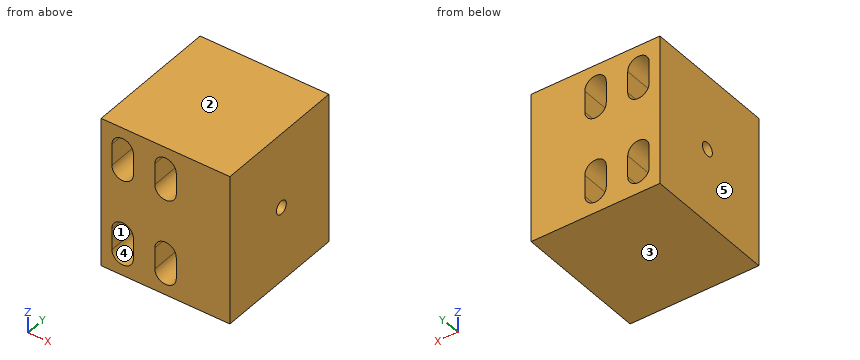
from build123d import *

# Parameters (mm, degrees)
SKETCH1_W           = 24
SKETCH1_H           = 28
BOSS_EXTRUDE1_DEPTH = 25
SKETCH2_R           = 1.25
CUT_EXTRUDE1_DEPTH  = 45.55333882


with BuildPart() as part:
    # Sketch1 → Boss-Extrude1 (new body)
    with BuildSketch(Plane(origin=(0, 0, 0), x_dir=(1, 0, 0), z_dir=(0, 1, 0))):
        with Locations((12, 14)):
            Rectangle(SKETCH1_W, SKETCH1_H)
        with BuildLine():
            Line((2, 4), (2, 8))
            ThreePointArc((2, 8), (4, 10), (6, 8))
            Line((6, 8), (6, 4))
            ThreePointArc((6, 4), (4, 2), (2, 4))
        make_face(mode=Mode.SUBTRACT)
        with BuildLine():
            Line((10, 4), (10, 8))
            ThreePointArc((10, 8), (12, 10), (14, 8))
            Line((14, 8), (14, 4))
            ThreePointArc((14, 4), (12, 2), (10, 4))
        make_face(mode=Mode.SUBTRACT)
        with BuildLine():
            Line((10, 20), (10, 24))
            ThreePointArc((10, 24), (12, 26), (14, 24))
            Line((14, 24), (14, 20))
            ThreePointArc((14, 20), (12, 18), (10, 20))
        make_face(mode=Mode.SUBTRACT)
        with BuildLine():
            Line((2, 20), (2, 24))
            ThreePointArc((2, 24), (4, 26), (6, 24))
            Line((6, 24), (6, 20))
            ThreePointArc((6, 20), (4, 18), (2, 20))
        make_face(mode=Mode.SUBTRACT)
    extrude(amount=BOSS_EXTRUDE1_DEPTH)

    # Sketch2 → Cut-Extrude1 (cut, through all)
    with BuildSketch(Plane(origin=(24, 0, 0), x_dir=(0, 0, -1), z_dir=(1, 0, 0))):
        with Locations((14, 13)):
            Circle(SKETCH2_R)
    extrude(amount=-CUT_EXTRUDE1_DEPTH, mode=Mode.SUBTRACT)


solid = part.part
For this review, take the finished solid that the model builds, in its own axes (mm). Face numbers are marked on the shaded views. A direction names the side the tool comes from. Coordinates: 2 decimals unless noted, no trailing zeros. Loops run counter-clockwise (first coordinate to the right, second up) from the corner with the lowest first, then second, coordinate; pieces in that order, holes last. Notation, with made-up numbers: (86.5, 17.5) - (92.5, 17.5) arc R14 ccw to (92.5, 37.5) - close; hole circle Ø10 at (69.25, 71). An arc over 180 degrees is marked (long way). Return JSON: item names as keys, results as strings.
Item 1: For the marked faces 1 and 2, list the 3-axis set-ups (+Z, -Z, +X, -X, +Y, -Y) from which the entire face can be reached by the end or side of a thin tool; tool diameter is ignored.
Determined:
{"face 1": "+Y, -Y", "face 2": "+Z, +X, -X, +Y, -Y"}
Item 2: Take a section at D-D (z = -19). Give the boundary of the cut face in (x, y), then the cut area to 3 significant figures.
Determined:
{"outline": "(0, 0) - (2.27, 0) - (2.27, 25) - (0, 25) - close; (5.73, 0) - (10.27, 0) - (10.27, 25) - (5.73, 25) - close; (13.73, 0) - (24, 0) - (24, 25) - (13.73, 25) - close", "area": "427 mm2"}
Item 3: Mouldability with a two-part tool opening along X and no side actions: class the marked faces 3, 4 and 5 as pulls with the +X half, pulls with the -X half, needs draft (parallel to the pull), parting line crosses it, or undercut.
Determined:
{"face 3": "needs draft", "face 4": "undercut", "face 5": "pulls with the -X half"}
Item 4: Take a section at B-B (x = 4). Give the boundary of the cut face in (y, z).
Determined:
{"outline": "(0, -28) - (25, -28) - (25, -26) - (0, -26) - close; (0, -18) - (25, -18) - (25, -10) - (0, -10) - close; (0, -2) - (25, -2) - (25, 0) - (0, 0) - close; hole circle Ø2.5 at (13, -14)"}
Item 5: Take a section at C-C (z = -14). Give the boundary of the cut face in (x, y).
Determined:
{"outline": "(0, 0) - (24, 0) - (24, 11.75) - (0, 11.75) - close; (0, 14.25) - (24, 14.25) - (24, 25) - (0, 25) - close"}
Item 6: For line 1 (X direction, y = 16.75, z = -6.5); line 2 (X direction, y = 8.5, z = -9.75); line 3 (Z direction, x = 3.5, y = 9.5), list the stretches that pass through material, from the lowest coordinate up.
Determined:
{"line 1": "x = 0 to 2, 6 to 10, 14 to 24", "line 2": "x = 0 to 3.03, 4.97 to 11.03, 12.97 to 24", "line 3": "z = -28 to -25.94, -18.06 to -9.94, -2.06 to 0"}
Item 7: Take a section at A-A (y = 13). Give the boundary of the cut face in (x, z).
Determined:
{"outline": "(0, -28) - (24, -28) - (24, -15.25) - (0, -15.25) - close; (0, -12.75) - (24, -12.75) - (24, 0) - (0, 0) - close; hole (2, -24) arc R2 ccw to (6, -24) - (6, -20) arc R2 ccw to (2, -20) - close; hole (2, -8) arc R2 ccw to (6, -8) - (6, -4) arc R2 ccw to (2, -4) - close; hole (10, -24) arc R2 ccw to (14, -24) - (14, -20) arc R2 ccw to (10, -20) - close; hole (10, -8) arc R2 ccw to (14, -8) - (14, -4) arc R2 ccw to (10, -4) - close"}
Item 8: Insertion check: pin 1 (3 mm diameter, centred on y = 3.5, z = -15, fed in from -X). The pin has a flat end and moves straight along its axis. Give the tip position at first contact, or say it passes through.
Determined:
{"pin 1": "stops at x = 0"}
